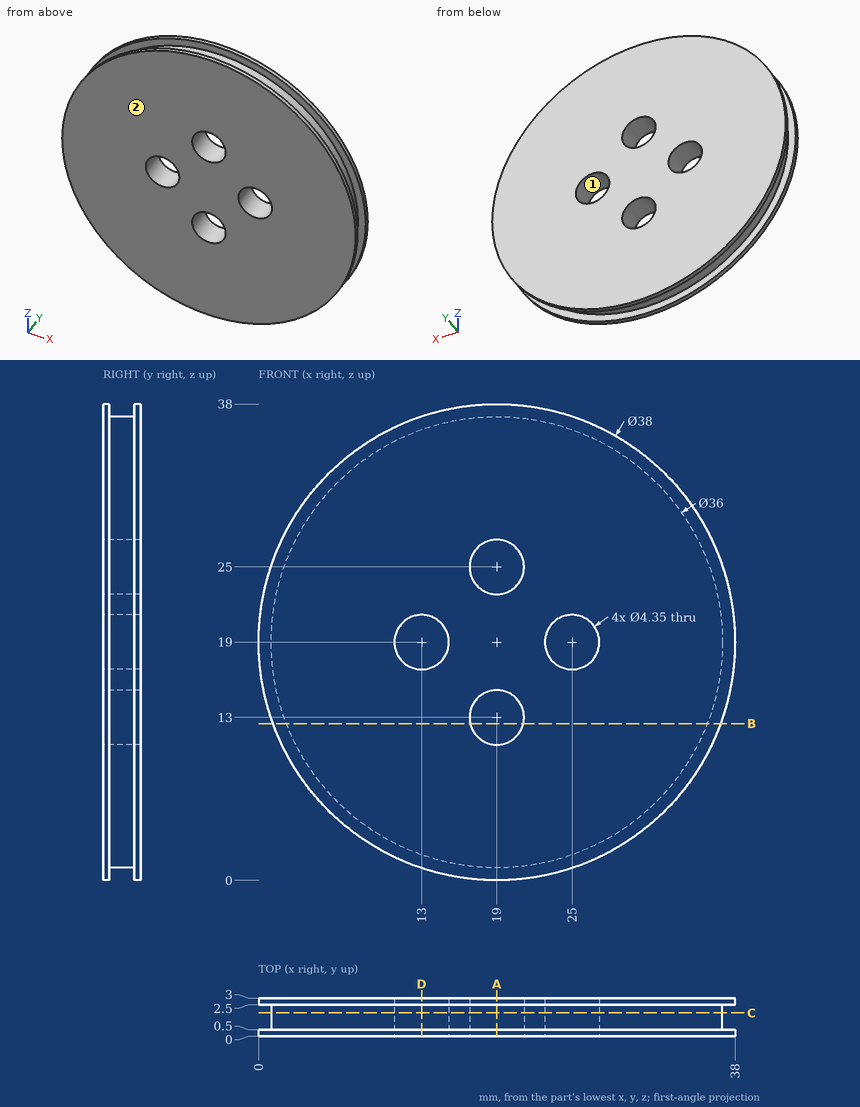
Drawing for the job (mm, zero at the part's lowest x, y, z). Give positions to 0.01 mm unless a question says otherwise; leave off trailing zeros. Loops run counter-clockwise (first coordinate to the right, second up) from the corner with the lowest first, then second, coordinate; pieces in that order, holes last. Notation, with made-up numbers: (49, 17.25) - (74, 17.25) arc R28 cw to (74, 41.25) - close; hole circle Ø7 at (65.25, -5). An arc over 180 degrees is marked (long way). Write item = value, one per line. Start each with the question number.
1) Band-saw the part on A-A on x = 19. Give the cut face in (y, z) (3 decimals).
2) Band-saw the part on D-D on x = 13. Give the cut face in (y, z) (3 decimals).
3) Pull direction Z, two halves, no side cores. Call the marked faces 1 and 2: +Z half, -Z half, draft (parallel to the pull), parting line (faces both ways), or undercut.
4) Band-saw the part on B-B on z = 12.5. Give the cut face in (x, y), plus the area to 3 significant figures.
5) Band-saw the part on C-C on y = 1.85. Give the cut face in (x, z) (3 decimals).
6) Probe probe 1 along Z at (x, y) = (19, 1.6) (3 decimals); probe 2 along X at (y, z) = (1.9, 17). List the from-to ranges inside material, lowest first. Write a range as from..to.
Final values:
q1.outline = (0, 0) - (0.5, 0) - (0.5, 1) - (2.5, 1) - (2.5, 0) - (3, 0) - (3, 10.825) - (0, 10.825) - close; (0, 15.175) - (3, 15.175) - (3, 22.825) - (0, 22.825) - close; (0, 27.175) - (3, 27.175) - (3, 38) - (2.5, 38) - (2.5, 37) - (0.5, 37) - (0.5, 38) - (0, 38) - close
q2.outline = (0, 0.972) - (0.5, 0.972) - (0.5, 2.029) - (2.5, 2.029) - (2.5, 0.972) - (3, 0.972) - (3, 16.825) - (0, 16.825) - close; (0, 21.175) - (3, 21.175) - (3, 37.028) - (2.5, 37.028) - (2.5, 35.971) - (0.5, 35.971) - (0.5, 37.028) - (0, 37.028) - close
q3.face_1 = undercut
q3.face_2 = draft
q4.outline = (1.15, 0) - (16.88, 0) - (16.88, 3) - (1.15, 3) - (1.15, 2.5) - (2.21, 2.5) - (2.21, 0.5) - (1.15, 0.5) - close; (21.12, 0) - (36.85, 0) - (36.85, 0.5) - (35.79, 0.5) - (35.79, 2.5) - (36.85, 2.5) - (36.85, 3) - (21.12, 3) - close
q4.area = 90.1 mm²
q5.outline = circle Ø36 at (19, 19); hole circle Ø4.35 at (13, 19); hole circle Ø4.35 at (19, 13); hole circle Ø4.35 at (19, 25); hole circle Ø4.35 at (25, 19)
q6.probe_1 = 1..10.825, 15.175..22.825, 27.175..37
q6.probe_2 = 1.11..12.15, 13.85..24.15, 25.85..36.89
